Check sheet for the modelled part. Datum: model origin and axes. Units: mm. Give positions to 0.01 mm unless a question says otherwise; leave off trailing zeros. Write each loop counter-clockwise with the first axis right and the second up, starting at its lowest first coordinate (ties: lowest second). Pieces come first, ordered by that corner, then holes. Notation, with made-up numbers: M -30,72.5 L -21,72.5 A19 ccw -21,106.5 Z; hole C -27.75,67.25 d4. An arc over 180 degrees is marked long. Write item = value, one per line. Start each with the question number.
1) Gauge pin test, flat ends, axial feed: pin 1 (1.9 mm diameter, centred on y = 492.5, z = 3.5, fed in from +X); pin 2 (3 mm diameter, centred on x = 12.5, z = 3, fed in from +Y); pin 3 (5 mm diameter, centred on x = 12.7, y = 12.7, fed in from -Z). Record the tip position at first contact, or that the pin passes through.
2) Scan lines: L1, parallel to X at y = 546.1, z = 2.5 (3 decimals); L2, parallel to Y at x = 38.1, z = 4 (3 decimals); L3, parallel to Y at x = 469.9, z = 4.25 (3 decimals). Record each from-to range of solid material in increasing order.
3) Sectioned sample at A-A, the plane z = 3.75. Record the cut outline in (x, y) (3 decimals), then the cut area to 3 significant figures.
4) Sectioned sample at B-B, the plane y = 431.5. Record the cut outline in (x, z).
Autodesk Inventor part; units mm, degrees
ref_plane "YZ Plane" through (0, 0, 0) normal (1, 0, 0) x (0, 1, 0)
ref_plane "XZ Plane" through (0, 0, 0) normal (0, 1, 0) x (-1, 0, 0)
ref_plane "XY Plane" through (0, 0, 0) normal (0, 0, 1) x (1, 0, 0)
sketch "Sketch1" plane through (0, 0, 0) normal (0, 0, 1) x (1, 0, 0)
  line L0 (0, 0) -> (482.6, 0)
  line L1 (482.6, 0) -> (482.6, 558.8)
  line L2 (482.6, 558.8) -> (0, 558.8)
  line L3 (0, 558.8) -> (0, 0)
  circle A0 centre (12.7, 12.7) radius 3.175
  circle A1 centre (469.9, 12.7) radius 3.175
  dimension "d0" = 558.8
  dimension "d1" = 482.6
  dimension "d2" = 6.35
  dimension "d3" = 6.35
  dimension "d4" = 12.7
  dimension "d5" = 12.7
  dimension "d7" = 12.7
  dimension "d8" = 12.7
extrude "Extrusion1" add sketch "Sketch1" along normal blind 6.35
sketch "Sketch2" plane through (0, 0, 0) normal (0, 0, -1) x (-1, 0, 0)
  line L0 (0, 558.8) -> (0, 0)
  line L1 (-482.6, 558.8) -> (0, 558.8)
  line L2 (-482.6, 0) -> (-482.6, 558.8)
  line L3 (-482.6, 558.8) -> (-457.2, 558.8)
  line L4 (-457.2, 558.8) -> (-457.2, 406.4)
  line L5 (-457.2, 406.4) -> (-482.6, 406.4)
  line L6 (-482.6, 406.4) -> (-482.6, 558.8)
  line L7 (0, 558.8) -> (-25.4, 558.8)
  line L8 (-25.4, 558.8) -> (-25.4, 406.4)
  line L9 (-25.4, 406.4) -> (0, 406.4)
  line L10 (0, 406.4) -> (0, 558.8)
  dimension "d13" = 25.4
  dimension "d16" = 152.4
extrude "Extrusion2" cut sketch "Sketch2" against normal through all
sketch "Sketch3" plane through (0, 0, 6.35) normal (0, 0, 1) x (1, 0, 0)
  line L0 (457.2, 406.4) -> (457.2, 558.8)
  line L1 (25.4, 558.8) -> (457.2, 558.8)
  line L2 (25.4, 558.8) -> (25.4, 406.4)
  circle A0 centre (38.1, 546.1) radius 3.175
  circle A1 centre (444.5, 546.1) radius 3.175
  dimension "d17" = 6.35
  dimension "d18" = 6.35
  dimension "d19" = 12.7
  dimension "d20" = 12.7
  dimension "d21" = 12.7
  dimension "d22" = 12.7
extrude "Extrusion3" cut sketch "Sketch3" against normal through all
properties part number "ElectronicsBoard" material "Wood (Birch)"
Data:
q1.pin_1 = 457.2
q1.pin_2 = 406.4
q1.pin_3 = through
q2.L1 = 25.4 to 34.925, 41.275 to 441.325, 447.675 to 457.2
q2.L2 = 0 to 542.925, 549.275 to 558.8
q2.L3 = 0 to 9.525, 15.875 to 406.4
q3.outline = M 0,0 L 482.6,0 L 482.6,406.4 L 457.2,406.4 L 457.2,558.8 L 25.4,558.8 L 25.4,406.4 L 0,406.4 Z; hole C 12.7,12.7 d6.35; hole C 38.1,546.1 d6.35; hole C 444.5,546.1 d6.35; hole C 469.9,12.7 d6.35
q3.area = 262,000 mm2
q4.outline = M 25.4,0 L 457.2,0 L 457.2,6.35 L 25.4,6.35 Z
